For this review, take the finished solid that the model builds, in its own axes (mm). Give positions to 0.01 mm unless a question says otherwise; leave off trailing zeros. Write each loop counter-clockwise with the first axis right and the second up, starting at its lowest first coordinate (ties: lowest second). Pieces come first, ordered by that corner, then holes. Notation, with made-up numbers: (-8.5, 27.25) -> (23.5, 27.25) arc R22 ccw to (23.5, 48.25) -> close; hole circle Ø9 at (74.25, -20.75). An arc over 180 degrees is marked (long way). Answer as CSV lines item,"result".
```python
from build123d import *

# Parameters (mm, degrees)
BOSS_EXTRU_1_DEPTH = 6
CONG_1_R           = 10


with BuildPart() as part:
    # Esquisse1 → Boss.-Extru.1 (new body)
    with BuildSketch(Plane.XY):
        Polygon((-176, 100), (-176, 0), (-92.57, -86.25), (92.57, -86.25), (176, 0), (176, 100), align=None)
    extrude(amount=BOSS_EXTRU_1_DEPTH)

    # Congé1
    cong_1_edges = [part.edges().sort_by_distance(p)[0] for p in [
        (176, 100, 3),
        (176, 0, 3),
        (92.57, -86.25, 3),
        (-92.57, -86.25, 3),
        (-176, 0, 3),
        (-176, 100, 3),
    ]]
    fillet(cong_1_edges, radius=CONG_1_R)


solid = part.part
```
Q1. Add section C-C (x = 145). Write out the cut boundary in (y, z), plus the area to 3 significant figures.
Answer block:
outline,"(-32.05, 0) -> (100, 0) -> (100, 6) -> (-32.05, 6) -> close"
area,"792 mm2"
Q2. To check wall thickness, follow probe 1 along Y at (x, z) = (-89.5, 4.4); probe 2 along X at (y, z) = (-51.5, 5.05); probe 3 along X at (y, z) = (-69.5, 5). State the ranges of each line that lie inside material, in increasing order. Write a range as [from, to].
Answer block:
probe 1,"y = [-86.18, 100]"
probe 2,"x = [-126.18, 126.18]"
probe 3,"x = [-108.77, 108.77]"
Q3. Add section B-B (y = -64). Write out the cut boundary in (x, z), plus the area to 3 significant figures.
Answer block:
outline,"(-114.09, 0) -> (114.09, 0) -> (114.09, 6) -> (-114.09, 6) -> close"
area,"1,370 mm2"
Q4. Add section A-A (z = 2.55). Write out the cut boundary in (x, y).
Answer block:
outline,"(-176, 4.05) arc R10 ccw to (-173.19, -2.91) -> (-95.52, -83.2) arc R10 ccw to (-88.33, -86.25) -> (88.33, -86.25) arc R10 ccw to (95.52, -83.2) -> (173.19, -2.91) arc R10 ccw to (176, 4.05) -> (176, 90) arc R10 ccw to (166, 100) -> (-166, 100) arc R10 ccw to (-176, 90) -> close"
Q5. Clearance check with flat-ended pins moving along their axes: pin 1 (1.5 mm diameter, centred on y = -66.5, z = 1, fed in from +X); pin 2 (3 mm diameter, centred on y = -52.5, z = 4.5, fed in from -X). State where each tip first meets the part, or that it passes through.
Answer block:
pin 1,"stops at x = 112.4"
pin 2,"stops at x = -126.67"
